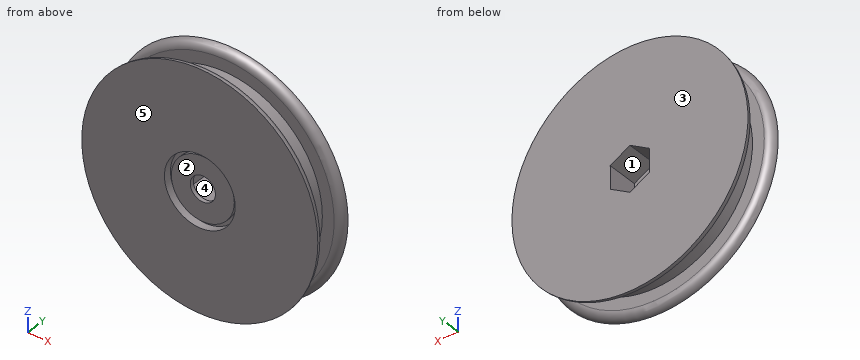
Autodesk Inventor part; units mm, degrees
ref_plane "YZ Plane" through (0, 0, 0) normal (1, 0, 0) x (0, 1, 0)
ref_plane "XZ Plane" through (0, 0, 0) normal (0, 1, 0) x (-1, 0, 0)
ref_plane "XY Plane" through (0, 0, 0) normal (0, 0, 1) x (1, 0, 0)
sketch "스케치1" plane through (0, 0, 0) normal (0, 1, 0) x (-1, 0, 0)
  line L0 (2.4971, 1.4484) -> (2.5029, -1.4383)
  line L1 (2.5029, -1.4383) -> (0.0058, -2.8867)
  line L2 (0.0058, -2.8867) -> (-2.4971, -1.4484)
  line L3 (-2.4971, -1.4484) -> (-2.5029, 1.4383)
  line L4 (-2.5029, 1.4383) -> (-0.0058, 2.8867)
  line L5 (-0.0058, 2.8867) -> (2.4971, 1.4484)
  circle A0 centre (0, 0) radius 4.5
  circle A1 centre (0, 0) radius 15
  circle A2 centre (0, 0) radius 12.5
  dimension "d0" = 5
  dimension "d1" = 9
  dimension "d2" = 30
  dimension "d3" = 25
extrude "돌출1" add sketch "스케치1" along normal blind 5 contours A0
sketch "스케치2" plane through (0, 0, 0) normal (0, -1, 0) x (1, 0, 0)
  circle A0 centre (0, 0) radius 15
  circle A1 centre (0, 0) radius 4.5
  dimension "d6" = 30
extrude "돌출2" add sketch "스케치2" along normal blind 1
sketch "스케치3" plane through (0, 0, 0) normal (0, 1, 0) x (1, 0, 0)
  circle A0 centre (0, 0) radius 12.5
  circle A1 centre (0, 0) radius 4.5
  dimension "d9" = 25
extrude "돌출3" add sketch "스케치3" along normal blind 3
sketch "스케치4" plane through (0, 3, 0) normal (0, 1, 0) x (1, 0, 0)
  circle A0 centre (0, 0) radius 15
  circle A1 centre (0, 0) radius 4.5
  dimension "d12" = 30
extrude "돌출4" add sketch "스케치4" along normal blind 1
fillet "모깎기1" radius 1 2 edges at (-15, 0, 0) (-15, 3, 0)
sketch "스케치5" plane through (0, 0, 0) normal (0, -1, 0) x (1, 0, 0)
  circle A0 centre (0, 0) radius 4
  line L0 (-0.0058, -2.8867) -> (-2.5029, -1.4383)
  line L1 (-2.5029, -1.4383) -> (-2.4971, 1.4484)
  line L2 (-2.4971, 1.4484) -> (0.0058, 2.8867)
  line L3 (0.0058, 2.8867) -> (2.5029, 1.4383)
  line L4 (2.5029, 1.4383) -> (2.4971, -1.4484)
  line L5 (2.4971, -1.4484) -> (-0.0058, -2.8867)
  circle A1 centre (0, 0) radius 4.5
  line L6 (-2.5029, -1.4383) -> (-2.4971, 1.4484)
  circle A2 centre (0, 0) radius 4.5
  dimension "d16" = 8
extrude "돌출5" add sketch "스케치5" along normal blind 0.5 contours A0 | L0 L1 L2 L3 L4 L5
sketch "스케치6" plane through (0, -0.5, 0) normal (0, -1, 0) x (1, 0, 0)
  circle A0 centre (0, 0) radius 1.6
  dimension "d19" = 3.2
extrude "돌출6" cut sketch "스케치6" against normal blind 0.5
sketch "스케치7" plane through (0.0058, 0, 2.8867) normal (-0.5017425, 0, -0.8650171) x (-0.8650171, 0, 0.5017425)
  point P0 (-1.4434, 0)
sketch "스케치8" plane through (0, -1, 0) normal (0, -1, 0) x (1, 0, 0)
  point P0 (0, 0)
sketch "스케치9" plane through (0, -1, 0) normal (0, -1, 0) x (1, 0, 0)
  line L0 (-2.5029, -1.4383) -> (-0.0058, -2.8867)
  line L1 (-0.0058, -2.8867) -> (2.4971, -1.4484)
  line L2 (2.4971, -1.4484) -> (2.5029, 1.4383)
  line L3 (2.5029, 1.4383) -> (0.0058, 2.8867)
  line L4 (0.0058, 2.8867) -> (-2.4971, 1.4484)
  line L5 (-2.4971, 1.4484) -> (-2.5029, -1.4383)
  circle A0 centre (0, 0) radius 4.5
  circle A1 centre (0, 0) radius 4.5
  circle A2 centre (0, 0) radius 15
  circle A3 centre (0, 0) radius 4.5
move faces "이동1" translate (0, -0.5, 0) faces at (-3.1667, 5, 0.0034) (-4.4417, 4.3333, -0.7219)
move faces "이동2" translate (0, -0.5, 0) faces at (-3.1667, 4.5, 0.0034)
sketch "스케치10" plane through (0.0058, 0, 2.8867) normal (-0.5017425, 0, -0.8650171) x (-0.8650171, 0, 0.5017425)
  point P0 (-1.4434, 0)
sketch "스케치11" plane through (0, 4, 0) normal (0, 1, 0) x (1, 0, 0)
  line L0 (-0.0058, 2.8867) -> (2.4971, 1.4484)
  line L1 (0.0058, -2.8867) -> (-2.4971, -1.4484)
  point P0 (0, 0)
  dimension "d28" = 5
properties part number "모터기어"
Geometry check sheet. Reference: the model listing, model coordinates, mm. Face numbers are marked on the shaded views. A direction names the side the tool comes from. Give positions to 0.01 mm unless a question says otherwise; leave off trailing zeros. Write each loop counter-clockwise with the first axis right and the second up, starting at its lowest first coordinate (ties: lowest second). Pieces come first, ordered by that corner, then holes.
1) Section check A-A, the plane y = 0.5. Record the boundary of the cut face in (x, z).
2) Access from +Z, -Z, +X, -X, +Y, -Y to the whole of each face (thin tool, end or side, straight path). Record for the marked faces 1, 2 and 3.
3) Gauge pin test, flat ends, axial feed: pin 1 (5.5 mm diameter, centred on x = 0, z = 0, fed in from -Y); pin 2 (1.5 mm diameter, centred on x = 1, z = 1, fed in from +Y). Record the tip position at first contact, or that the pin passes through.
4) Section check C-C, the plane y = 3.55. Record the boundary of the cut face in (x, z), and give its area (3 significant figures).
5) Material ranges on L1, parallel to Y at x = -12.25, z = -4.5; L2, parallel to Z at x = 0, y = -0.3; L3, parallel to Z at x = 0, y = -0.15, recorded low to high.
6) Release check for a two-part mould opening along X. For the marked faces 4 and 5 record: pulls with the +X half, pulls with the -X half, needs draft (parallel to the pull), parting line crosses it, or undercut.
Computed:
1. outline: circle Ø25 at (0, 0); hole (-2.5, -1.44) - (-0.01, -2.89) - (2.5, -1.45) - (2.5, 1.44) - (0.01, 2.89) - (-2.5, 1.45) - close
2. face 1: +Y
2. face 2: -Y
2. face 3: +Z, -Z, +X, -X, +Y
3. pin 1: stops at y = -0.5
3. pin 2: stops at y = 0
4. outline: circle Ø29.79 at (0, 0); hole (-2.5, -1.44) - (-0.01, -2.89) - (2.5, -1.45) - (2.5, 1.44) - (0.01, 2.89) - (-2.5, 1.45) - close
4. area: 675 mm2
5. L1: y = -1 to 0, 3 to 4
5. L2: z = -14.71 to -4.5, -4 to -1.6, 1.6 to 4, 4.5 to 14.71
5. L3: z = -14.53 to -4.5, -4 to -1.6, 1.6 to 4, 4.5 to 14.53
6. face 4: undercut
6. face 5: needs draft
